Drawing for the job (mm, zero at the part's lowest x, y, z). Give positions to 0.01 mm unless a question says otherwise; leave off trailing zeros. Loops run counter-clockwise (first coordinate to the right, second up) from the corner with the lowest first, then second, coordinate; pieces in that order, holes last.
1) Band-saw the part on A-A on z = 13. State how many separate pieces and enclosed holes the cut face has, then the cut area to 3 significant figures.
2) Two-plate mould, pull along X, no slides. Class the marked faces 1, 2 and 3: +X half, -X half, draft (parallel to the pull), parting line (faces both ways), or undercut.
3) Band-saw the part on B-B on x = 106. List the corners of the cut face in (y, z) (1 decimal), then the cut area to 3 significant figures.
4) Flat gauge pin, fed straight in: P1, Ø13.5, axis at x = 15.875, z = 19.05, coming from the -Y side. Where does the tip first touch, or does it go through?
5) Wall check: line 1 (X direction, y = 73, z = 21); line 2 (Z direction, x = 40.5, y = 18); line 3 (Z direction, x = 15, y = 47). Give the ranges that are in metal, low to high.
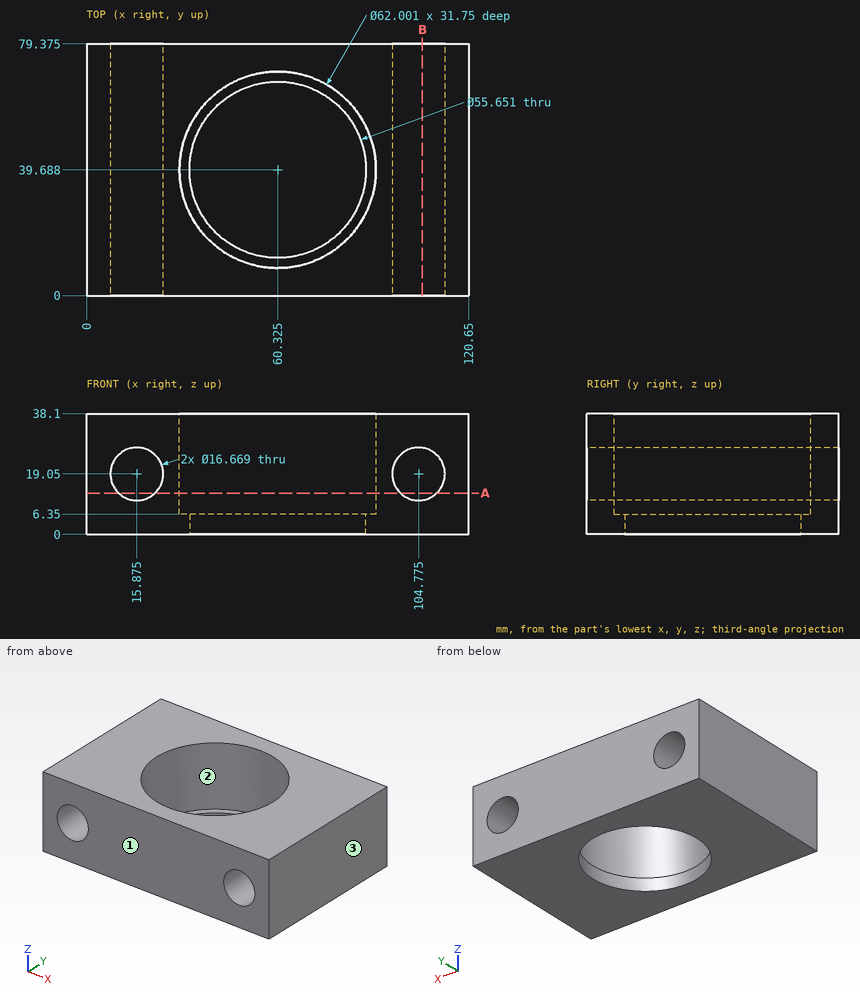
Findings below:
1. separate pieces: 3
1. enclosed holes: 1
1. area: 4,740 mm2
2. face 1: draft
2. face 2: undercut
2. face 3: +X half
3. outline: (0, 0) - (79.4, 0) - (79.4, 10.8) - (0, 10.8) - close; (0, 27.3) - (79.4, 27.3) - (79.4, 38.1) - (0, 38.1) - close
3. area: 1,720 mm2
4. P1: passes through
5. line 1: x = 0 to 7.77, 23.98 to 96.67, 112.88 to 120.65
5. line 2: z = 0 to 6.35
5. line 3: z = 0 to 10.76, 27.34 to 38.1
